Work out the finished part from the listing and answer in its coordinate system (mm). A direction names the side the tool comes from. Round coordinates to 2 decimals unless told otherwise and drop trailing zeros. Write each loop counter-clockwise with the first axis right and the second up, starting at its lowest first coordinate (ties: lowest second). Pieces come first, ordered by that corner, then holes. Notation, with made-up numbers: (-17, 10) - (4, 10) arc R35 ccw to (4, 46) - close; hole circle Ø7 at (32, -34.5). An arc over 180 degrees is marked (long way). Answer as a JSON object with one key per item and string values.
Autodesk Fusion 360 part; units mm, degrees
sketch "Sketch1" plane through (0, 0, 0) normal (0, 1, 0) x (1, 0, 0)
  circle A0 centre (0, 0) radius 32
  circle A1 centre (0, 100) radius 24
  line L0 (32, 0) -> (32, 10)
  line L1 (32, 10) -> (23.9079, 102.1006)
  line L2 (-31.9991, 0.2374) -> (-23.9247, 101.9002)
  dimension "d1" = 64
  dimension "d2" = 48
extrude "Extrude1" add sketch "Sketch1" along normal blind 12 contours A0 A1 L0 L1 L2 makes body 1
sketch "Sketch2" plane through (0, 12, 0) normal (0, 1, 0) x (-1, 0, 0)
  line L0 (-32, -10) -> (-23.9079, -102.1006)
  arc A0 (23.9247, -101.9002) -> (-23.9079, -102.1006) centre (0, -100) ccw
  line L1 (23.9247, -101.9002) -> (31.6354, -4.8167)
  arc A1 (-32, 0) -> (31.6354, -4.8167) centre (0, 0) ccw
  line L2 (-32, 0) -> (-32, -10)
  circle A2 centre (0, 0) radius 32
  circle A3 centre (0, 0) radius 18
extrude "Extrude2" add sketch "Sketch2" against normal blind 36 contours A1 A2 bodies 1
sketch "Sketch3" plane through (0, 12, 0) normal (0, 1, 0) x (-1, 0, 0)
  circle A0 centre (0, 0) radius 18
  line L0 (-32, -10) -> (-23.9079, -102.1006)
  arc A1 (23.9247, -101.9002) -> (-23.9079, -102.1006) centre (0, -100) ccw
  line L1 (23.9247, -101.9002) -> (31.6354, -4.8167)
  arc A2 (31.6354, -4.8167) -> (-32, 0) centre (0, 0) ccw
  line L2 (-32, 0) -> (-32, -10)
  circle A3 centre (0, -100) radius 24
  circle A4 centre (0, -100) radius 12
  dimension "d7" = 24
extrude "Extrude3" add sketch "Sketch3" against normal blind 24 contours A1 A3 bodies 1
sketch "Sketch4" plane through (0, 12, 0) normal (0, 1, 0) x (-1, 0, 0)
  circle A0 centre (0, -100) radius 12
  circle A1 centre (0, 0) radius 18
  line L0 (-32, -10) -> (-23.9079, -102.1006)
  arc A2 (-23.9079, -102.1006) -> (23.9247, -101.9002) centre (0, -100) ccw
  line L1 (23.9247, -101.9002) -> (31.6354, -4.8167)
  arc A3 (31.6354, -4.8167) -> (-32, 0) centre (0, 0) ccw
  line L2 (-32, 0) -> (-32, -10)
  line L3 (-5.7314, -17.0631) -> (6, -17.0631)
  line L4 (6, -17.0631) -> (6, -23)
  line L5 (6, -23) -> (-5.7314, -23)
  line L6 (-5.7314, -23) -> (-5.7314, -17.0631)
extrude "Extrude4" cut sketch "Sketch4" against normal blind 36 contours A1 L3 L4 L5 L6 bodies 1
sketch "Sketch5" plane through (0, 0, 0) normal (1, 0, 0) x (0, 1, 0)
  line L0 (-12, -76) -> (-24, -32)
  line L1 (-24, -32) -> (0, -32)
  line L2 (0, -32) -> (0, -76)
  line L3 (0, -76) -> (-12, -76)
extrude "Extrude5" add sketch "Sketch5" along normal blind 6 separate body makes body 2
sketch "Sketch6" plane through (0, 0, 0) normal (-1, 0, 0) x (0, -1, 0)
  line L0 (0, -32) -> (0, -76)
  line L1 (0, -76) -> (12, -76)
  line L2 (12, -76) -> (24, -32)
  line L3 (24, -32) -> (0, -32)
  line L4 (24, -32) -> (0, -32)
  line L5 (0, -76) -> (12, -76)
extrude "Extrude6" add sketch "Sketch6" along normal blind 6 bodies 2 1
sketch "Sketch7" plane through (0, 0, 0) normal (0, 0, 1) x (1, 0, 0)
  spline S0 degree 5 poles (-200, -70) (-199.5071, -70.1071) (-198.5439, -70.3047) (-197.1668, -70.5516) (-195.4683, -70.7802) (-193.5919, -70.8856) (-191.9888, -70.7912) (-190.6902, -70.4741) (-189.725, -69.9134) (-189.1054, -69.1001) (-188.8176, -68.0441) (-188.8364, -67.0173) (-188.9827, -66.1506) (-189.138, -65.5306) (-189.2301, -65.21) knots 0 0 0 0 0 0 0.1 0.2 0.3 0.4 0.5 0.6 0.7 0.8 0.9 1 1 1 1 1 1
  point P0 (-190, -70)
Item 1: Determine the mould class of faces 5 (the flat face through (0, 12, -45)), 6 (the cylindrical face through (-0.71, -5.748, 17.986)), 7 (the flat face through (-4, -12, -32)) for opening direction Y: pulls with the +Y half, pulls with the -Y half, needs draft (parallel to the pull), parting line crosses it, or undercut.
Results found:
{"face 5": "pulls with the +Y half", "face 6": "needs draft", "face 7": "undercut"}
Item 2: For faces 1 (the flat face through (4, -12, -32)), 2 (the flat face through (-14, -24, -14)), 3 (the flat face through (0, -6, -23)), 4 (the flat face through (-6, -9, -54)), determine the directions among +Z, -Z, +X, -X, +Y, -Y from which every point of the face is accessible in a straight line to the end or side of a thin tool.
Results found:
{"face 1": "none", "face 2": "+Z, -Z, +X, -X, -Y", "face 3": "+Y, -Y", "face 4": "-X, -Y"}
Item 3: A cutting plane is placed at C-C (x = -3.5). Write down the section's boundary in (y, z), and give its area (3 significant figures).
Results found:
{"outline": "(-24, -32) - (-12, -76) - (0, -76) - (0, -76.26) - (-12, -76.26) - (-12, -88.52) - (12, -88.52) - (12, -23) - (-24, -23) - (-24, -31.81) - (0, -31.81) - (0, -32) - close; (-24, 17.66) - (12, 17.66) - (12, 31.81) - (-24, 31.81) - close; (-12, -123.74) - (12, -123.74) - (12, -111.48) - (-12, -111.48) - close", "area": "2,740 mm²"}
Item 4: Consider line 1 along Z through (x, y) = (0, 4.5); line 2 along X through (y, z) = (-10, 0); line 3 along Z through (x, y) = (10, -6.5). Determine where each line is inside the solid, lowest interval first.
Results found:
{"line 1": "-124 to -112, -88 to -23, 18 to 32", "line 2": "-32 to -18, 18 to 32", "line 3": "-121.82 to -106.63, -93.37 to -78.18, -30.4 to -14.97, 14.97 to 30.4"}
Item 5: A cutting plane is placed at B-B (z = -100). Write down the section's boundary in (x, y).
Results found:
{"outline": "(-24.08, 0) - (-24, 0) - (-24, -12) - (-12, -12) - (-12, 12) - (-24.08, 12) - close; (12, -12) - (24, -12) - (24, 0) - (24.09, 0) - (24.09, 12) - (12, 12) - close"}
Item 6: Each of these flat-tipped pins is pushed along its axis until it touches: P1, Ø6.5, axis at x = 4, y = -6, coming from the -Z side; P2, Ø9.5, axis at x = 1, y = -1.5, coming from the +Z side; P3, Ø1, axis at x = -24, y = -3.5, coming from the +Z side; P4, Ø19, axis at x = 0, z = -100, coming from the -Y side. Where does it stop, or does it pass through?
Results found:
{"P1": "z = -123.99", "P2": "z = 32", "P3": "z = 21.72", "P4": "through"}
